Source: CAD feature listing. Evaluate the final solid. Frame: model axes, mm. Coordinates: 2 decimals unless noted, no trailing zeros. Order: outer loops, then holes, each group sorted by start corner. A loop starts at its lowest first (then second) coordinate and runs counter-clockwise, first axis right, second up.
```python
from build123d import *

# Parameters (mm, degrees)
F0_W      = 400
F0_H      = 12
F1_DEPTH  = 450
F2_W      = 40
F2_H      = 60
F3_DEPTH  = 12
F4_W      = 40
F4_H      = 60
F5_DEPTH  = 15
F6_W      = 40
F6_H      = 60
F7_DEPTH  = 15
F8_W      = 40
F8_H      = 60
F9_DEPTH  = 15
F10_R     = 3
F11_DEPTH = 12
F12_R     = 3
F13_DEPTH = 12
F14_R     = 3
F15_DEPTH = 12
F16_R     = 3
F17_DEPTH = 12


with BuildPart() as f1:
    # F0 (on Front) → F1 (new body, symmetric)
    with BuildSketch(Plane.XZ):
        with Locations((200, 6)):
            Rectangle(F0_W, F0_H)
    extrude(amount=F1_DEPTH, both=True)

    # F2 (on face) → F3 (cut)
    with BuildSketch(Plane.XY.offset(12)):
        with Locations((20, 420)):
            Rectangle(F2_W, F2_H)
    extrude(amount=-F3_DEPTH, mode=Mode.SUBTRACT)

    # F4 (on face) → F5 (cut)
    with BuildSketch(Plane.XY.offset(12)):
        with Locations((380, 420)):
            Rectangle(F4_W, F4_H)
    extrude(amount=-F5_DEPTH, mode=Mode.SUBTRACT)

    # F6 (on face) → F7 (cut)
    with BuildSketch(Plane.XY.offset(12)):
        with Locations((380, -420)):
            Rectangle(F6_W, F6_H)
    extrude(amount=-F7_DEPTH, mode=Mode.SUBTRACT)

    # F8 (on face) → F9 (cut)
    with BuildSketch(Plane.XY.offset(12)):
        with Locations((20, -420)):
            Rectangle(F8_W, F8_H)
    extrude(amount=-F9_DEPTH, mode=Mode.SUBTRACT)

    # F10 (on face) → F11 (cut)
    with BuildSketch(Plane.XZ.offset(390)):
        with Locations((20, 6)):
            Circle(F10_R)
    extrude(amount=-F11_DEPTH, mode=Mode.SUBTRACT)

    # F12 (on face) → F13 (cut)
    with BuildSketch(Plane.XZ.offset(390)):
        with Locations((380, 6)):
            Circle(F12_R)
    extrude(amount=-F13_DEPTH, mode=Mode.SUBTRACT)

    # F14 (on face) → F15 (cut)
    with BuildSketch(Plane(origin=(0, 390, 0), x_dir=(-1, 0, 0), z_dir=(0, 1, 0))):
        with Locations((-380, 6)):
            Circle(F14_R)
    extrude(amount=-F15_DEPTH, mode=Mode.SUBTRACT)

    # F16 (on face) → F17 (cut)
    with BuildSketch(Plane(origin=(0, 390, 0), x_dir=(-1, 0, 0), z_dir=(0, 1, 0))):
        with Locations((-20, 6)):
            Circle(F16_R)
    extrude(amount=-F17_DEPTH, mode=Mode.SUBTRACT)


solid = f1.part
```
Q1. Material intervals for line 1 along Z through (x, y) = (20, -384.5); line 2 along Y through (x, z) = (37.5, 9.25); line 3 along X through (y, z) = (-393, 10.25), sorted ascending.
Solutions:
line 1: z = 0 to 3, 9 to 12
line 2: y = -390 to 390
line 3: x = 40 to 360
Q2. Pin query (flat end, axial travel): P1, Ø1.8, axis at x = 380, z = 6.5, coming from the +Y side; P2, Ø7, axis at x = 380, z = 6, coming from the +Y side; P3, Ø3, axis at x = 379, z = 6, coming from the -Y side; P4, Ø1.5, axis at x = 46.5, y = 76, coming from the -Z side. Return the tip coordinate at first contact, or that it passes through.
Solutions:
P1: stops at y = 378
P2: stops at y = 390
P3: stops at y = -378
P4: stops at z = 0
Q3. Section query A-A on z = 6. Output: boundary loops of the cut face in (x, y).
Solutions:
outline: (0, -390) - (17, -390) - (17, -378) - (23, -378) - (23, -390) - (40, -390) - (40, -450) - (360, -450) - (360, -390) - (377, -390) - (377, -378) - (383, -378) - (383, -390) - (400, -390) - (400, 390) - (383, 390) - (383, 378) - (377, 378) - (377, 390) - (360, 390) - (360, 450) - (40, 450) - (40, 390) - (23, 390) - (23, 378) - (17, 378) - (17, 390) - (0, 390) - close
